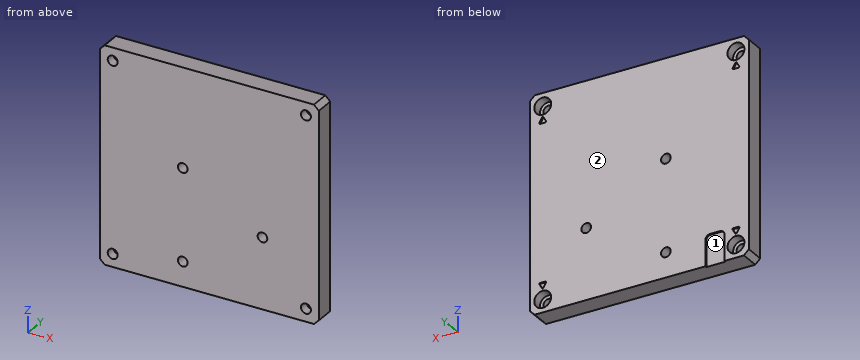
```python
from build123d import *

# Parameters (mm, degrees)
SKETCH_2_W             = 136
SKETCH_2_H             = 134
SKETCH_2_R             = 3.1
SKETCH_2_R_2           = 3
EXTRUDE_1_DEPTH        = 12
SKETCH_3_R             = 5.25
CUT_EXTRUDE_1165_DEPTH = 6
SKETCH_4_W             = 12
SKETCH_4_H             = 20
CUT_EXTRUDE_2_DEPTH    = 1
CHAMFER_1_SIZE         = 3
FILLET_1_R             = 3


with BuildPart() as part:
    # ｽｹｯﾁ2 → ﾎﾞｽ - 押し出し1 (new body)
    with BuildSketch(Plane(origin=(0, 0, 0), x_dir=(1, 0, 0), z_dir=(0, 1, 0))):
        with Locations((0, -23)):
            Rectangle(SKETCH_2_W, SKETCH_2_H)
        with Locations(Location((-60, 36, 0), (0, 0, 270))):
            Circle(SKETCH_2_R, mode=Mode.SUBTRACT)
        with Locations(Location((60, 36, 0), (0, 0, 270))):
            Circle(SKETCH_2_R, mode=Mode.SUBTRACT)
        with Locations(Location((60, -82, 0), (0, 0, 270))):
            Circle(SKETCH_2_R, mode=Mode.SUBTRACT)
        with Locations(Location((-60, -82, 0), (0, 0, 270))):
            Circle(SKETCH_2_R, mode=Mode.SUBTRACT)
        with Locations(Location((-16.5, 28.578838325, 0), (0, 0, 270))):
            Circle(SKETCH_2_R_2, mode=Mode.SUBTRACT)
        with Locations(Location((-16.5, -28.578838325, 0), (0, 0, 270))):
            Circle(SKETCH_2_R_2, mode=Mode.SUBTRACT)
        with Locations(Location((33, 0, 0), (0, 0, 270))):
            Circle(SKETCH_2_R_2, mode=Mode.SUBTRACT)
    extrude(amount=EXTRUDE_1_DEPTH)

    # ｽｹｯﾁ3 → Cut-Extrude 1165 (cut)
    with BuildSketch(Plane(origin=(0, 12, 0), x_dir=(1, 0, 0), z_dir=(0, 1, 0))):
        with Locations(Location((-60, 36, 0), (0, 0, 270))):
            Circle(SKETCH_3_R)
        with Locations(Location((60, 36, 0), (0, 0, 270))):
            Circle(SKETCH_3_R)
        with Locations(Location((-60, -82, 0), (0, 0, 270))):
            Circle(SKETCH_3_R)
        with Locations(Location((60, -82, 0), (0, 0, 270))):
            Circle(SKETCH_3_R)
    extrude(amount=-CUT_EXTRUDE_1165_DEPTH, mode=Mode.SUBTRACT)

    # ｽｹｯﾁ4 → ｶｯﾄ - 押し出し2 (cut)
    with BuildSketch(Plane(origin=(0, 12, 0), x_dir=(1, 0, 0), z_dir=(0, 1, 0))):
        with BuildLine():
            Line((57.933012702, 26.306624327), (59.566987298, 29.136751346))
            ThreePointArc((59.566987298, 29.136751346), (60, 29.386751346), (60.433012702, 29.136751346))
            Line((60.433012702, 29.136751346), (62.066987298, 26.306624327))
            ThreePointArc((62.066987298, 26.306624327), (62.066987298, 25.806624327), (61.633974596, 25.556624327))
            Line((61.633974596, 25.556624327), (58.366025404, 25.556624327))
            ThreePointArc((58.366025404, 25.556624327), (57.933012702, 25.806624327), (57.933012702, 26.306624327))
        make_face()
        with BuildLine():
            Line((-60.433012702, 29.136751346), (-62.066987298, 26.306624327))
            ThreePointArc((-62.066987298, 26.306624327), (-62.066987298, 25.806624327), (-61.633974596, 25.556624327))
            Line((-61.633974596, 25.556624327), (-58.366025404, 25.556624327))
            ThreePointArc((-58.366025404, 25.556624327), (-57.933012702, 25.806624327), (-57.933012702, 26.306624327))
            Line((-57.933012702, 26.306624327), (-59.566987298, 29.136751346))
            ThreePointArc((-59.566987298, 29.136751346), (-60, 29.386751346), (-60.433012702, 29.136751346))
        make_face()
        with BuildLine():
            Line((60.433012702, -75.136751346), (62.066987298, -72.306624327))
            ThreePointArc((62.066987298, -72.306624327), (62.066987298, -71.806624327), (61.633974596, -71.556624327))
            Line((61.633974596, -71.556624327), (58.366025404, -71.556624327))
            ThreePointArc((58.366025404, -71.556624327), (57.933012702, -71.806624327), (57.933012702, -72.306624327))
            Line((57.933012702, -72.306624327), (59.566987298, -75.136751346))
            ThreePointArc((59.566987298, -75.136751346), (60, -75.386751346), (60.433012702, -75.136751346))
        make_face()
        with BuildLine():
            Line((-57.933012702, -72.306624327), (-59.566987298, -75.136751346))
            ThreePointArc((-59.566987298, -75.136751346), (-60, -75.386751346), (-60.433012702, -75.136751346))
            Line((-60.433012702, -75.136751346), (-62.066987298, -72.306624327))
            ThreePointArc((-62.066987298, -72.306624327), (-62.066987298, -71.806624327), (-61.633974596, -71.556624327))
            Line((-61.633974596, -71.556624327), (-58.366025404, -71.556624327))
            ThreePointArc((-58.366025404, -71.556624327), (-57.933012702, -71.806624327), (-57.933012702, -72.306624327))
        make_face()
        with Locations((-47, 35)):
            Rectangle(SKETCH_4_W, SKETCH_4_H)
    extrude(amount=-CUT_EXTRUDE_2_DEPTH, mode=Mode.SUBTRACT)

    # 面取り1
    chamfer_1_edges = [part.edges().sort_by_distance(p)[0] for p in [
        (-68, 6, -44),
        (68, 6, -44),
        (68, 6, 90),
        (-68, 6, 90),
    ]]
    chamfer(chamfer_1_edges, length=CHAMFER_1_SIZE)

    # ﾌｨﾚｯﾄ1
    fillet_1_edges = [part.edges().sort_by_distance(p)[0] for p in [
        (-53, 11.5, -25),
        (-41, 11.5, -25),
    ]]
    fillet(fillet_1_edges, radius=FILLET_1_R)


solid = part.part
```
Check sheet for the modelled part. Datum: model origin and axes. Units: mm. Face numbers are marked on the shaded views. Round coordinates to 2 decimals unless told otherwise and drop trailing zeros. Loops run counter-clockwise (first coordinate to the right, second up) from the corner with the lowest first, then second, coordinate; pieces in that order, holes last. Notation, with made-up numbers: M 40.25,-14.5 L 56.25,-14.5 A14 cw 56.25,10.5 Z; hole C 52.25,44 d10. An arc over 180 degrees is marked long. Answer as a JSON object with one key per item and string values.
1. Section check B-B (y = 8.5). Record the boundary of the cut face in (x, z).
Reply:
{"outline": "M -68,-41 L -65,-44 L 65,-44 L 68,-41 L 68,87 L 65,90 L -65,90 L -68,87 Z; hole C -60,-36 d10.5; hole C -60,82 d10.5; hole C -16.5,-28.58 d6; hole C -16.5,28.58 d6; hole C 33,0 d6; hole C 60,-36 d10.5; hole C 60,82 d10.5"}
2. Scan lines: line 1 (X direction, y = 8.05, z = -36); line 2 (X direction, y = 1.5, z = 82); line 3 (Z direction, x = -17.5, y = 10.5). Record each from-to range of solid material in increasing order.
Reply:
{"line 1": "x = -68 to -65.25, -54.75 to 54.75, 65.25 to 68", "line 2": "x = -68 to -63.1, -56.9 to 56.9, 63.1 to 68", "line 3": "z = -44 to -31.41, -25.75 to 25.75, 31.41 to 90"}
3. Gauge pin test, flat ends, axial feed: P1, Ø6.5, axis at x = -60, z = -36, coming from the +Y side; P2, Ø1.1, axis at x = 60, z = -27, coming from the +Y side. Record the tip position at first contact, or that the pin passes through.
Reply:
{"P1": "stops at y = 6", "P2": "stops at y = 11"}
4. Mould release check, pull along X, two halves, no side actions. Record for the marked faces 1 and 2: pulls with the +X half, pulls with the -X half, needs draft (parallel to the pull), parting line crosses it, or undercut.
Reply:
{"face 1": "undercut", "face 2": "needs draft"}
5. Section check A-A (z = 82). Record the boundary of the cut face in (x, y), plus the area to 3 significant figures.
Reply:
{"outline": "M -68,0 L -63.1,0 L -63.1,6 L -65.25,6 L -65.25,12 L -68,12 Z; M -56.9,0 L 56.9,0 L 56.9,6 L 54.75,6 L 54.75,12 L -54.75,12 L -54.75,6 L -56.9,6 Z; M 63.1,0 L 68,0 L 68,12 L 65.25,12 L 65.25,6 L 63.1,6 Z", "area": "1,430 mm²"}
6. Section check C-C (z = -36). Record the boundary of the cut face in (x, y).
Reply:
{"outline": "M -68,0 L -63.1,0 L -63.1,6 L -65.25,6 L -65.25,12 L -68,12 Z; M -56.9,0 L 56.9,0 L 56.9,6 L 54.75,6 L 54.75,12 L -41,12 L -41,11 L -53,11 L -53,12 L -54.75,12 L -54.75,6 L -56.9,6 Z; M 63.1,0 L 68,0 L 68,12 L 65.25,12 L 65.25,6 L 63.1,6 Z"}
7. Section check D-D (z = 30). Record the boundary of the cut face in (x, y).
Reply:
{"outline": "M -68,0 L -19.14,0 L -19.14,12 L -68,12 Z; M -13.86,0 L 68,0 L 68,12 L -13.86,12 Z"}
